from build123d import *

# Parameters (mm, degrees)
PAD_DEPTH       = 12
SKETCH004_R     = 8
SKETCH004_R_2   = 1.25
PAD001_DEPTH    = 5
SKETCH005_R     = 1.25
POCKET_DEPTH    = 8
PAD002_DEPTH    = 2
FILLET_R        = 2
CHAMFER_SIZE    = 0.6
CHAMFER001_SIZE = 0.5
FILLET001_R     = 2
FILLET002_R     = 2
CHAMFER002_SIZE = 0.6


with BuildPart() as part:
    # Sketch002 → Pad (new body)
    with BuildSketch(Plane.XY):
        with BuildLine():
            ThreePointArc((0, -7.5), (4.245918, -6.182409), (7, -2.692582))
            Line((7, 2.692582), (7, -2.692582))
            ThreePointArc((7, 2.692582), (4.245918, 6.182409), (0, 7.5))
            Line((-10.65, 5.289572), (0, 7.5))
            Line((-10.65, 5.289572), (-10.65, -5.289572))
            Line((-10.65, -5.289572), (0, -7.5))
        make_face()
        with BuildLine():
            ThreePointArc((-2.65, -1.702939), (3.15, 0), (-2.65, 1.702939))
            Line((-2.65, 1.702939), (-2.65, -1.702939))
        make_face(mode=Mode.SUBTRACT)
    extrude(amount=PAD_DEPTH)

    # Sketch004 → Pad001 (join)
    with BuildSketch(Plane.XY.offset(12)):
        with BuildLine():
            Line((-10.65, 8.5), (57.640793, 8.5))
            ThreePointArc((57.640793, -8.5), (85, 0), (57.640793, 8.5))
            Line((57.640793, -8.5), (-10.65, -8.5))
            Line((-10.65, -8.5), (-10.65, 8.5))
        make_face()
        with Locations((70, 0)):
            Circle(SKETCH004_R, mode=Mode.SUBTRACT)
        with Locations((64.25, 9.959292)):
            Circle(SKETCH004_R_2, mode=Mode.SUBTRACT)
        with Locations((81.5, 0)):
            Circle(SKETCH004_R_2, mode=Mode.SUBTRACT)
        with Locations((64.25, -9.959292)):
            Circle(SKETCH004_R_2, mode=Mode.SUBTRACT)
        with BuildLine():
            ThreePointArc((-2.65, -1.702939), (3.15, 0), (-2.65, 1.702939))
            Line((-2.65, 1.702939), (-2.65, -1.702939))
        make_face(mode=Mode.SUBTRACT)
    extrude(amount=PAD001_DEPTH)

    # Sketch005 (on Face1 of Pad001) → Pocket (cut)
    with BuildSketch(Plane(origin=(-10.65, 0, 0), x_dir=(0, -1, 0), z_dir=(-1, 0, 0))):
        with Locations((0, 14.5)):
            Circle(SKETCH005_R)
        with Locations((0, 8.5)):
            Circle(SKETCH005_R)
        with Locations((0, 2.5)):
            Circle(SKETCH005_R)
    extrude(amount=-POCKET_DEPTH, mode=Mode.SUBTRACT)

    # Sketch006 (on Face16 of Pocket) → Pad002 (join, symmetric)
    with BuildSketch(Plane(origin=(0, 0, 0), x_dir=(-1, 0, 0), z_dir=(0, 1, 0))):
        Polygon((-7, 0), (-55, 12), (-7, 12), align=None)
    extrude(amount=PAD002_DEPTH, both=True)

    # Fillet
    fillet_edges = [part.edges().sort_by_distance(p)[0] for p in [
        (-10.65, 8.5, 14.5),
        (-10.65, 5.289572, 6),
        (-10.65, -5.289572, 6),
        (-10.65, -8.5, 14.5),
    ]]
    fillet(fillet_edges, radius=FILLET_R)

    # Chamfer
    chamfer_edges = [part.edges().sort_by_distance(p)[0] for p in [
        (3.15, 0, 0),
        (-2.65, 0, 0),
    ]]
    chamfer(chamfer_edges, length=CHAMFER_SIZE)

    # Chamfer001
    chamfer001_edges = [part.edges().sort_by_distance(p)[0] for p in [
        (62, 0, 12),
    ]]
    chamfer(chamfer001_edges, length=CHAMFER001_SIZE)

    # Fillet001
    fillet001_edges = [part.edges().sort_by_distance(p)[0] for p in [
        (57.640793, 8.5, 14.5),
    ]]
    fillet(fillet001_edges, radius=FILLET001_R)

    # Fillet002
    fillet002_edges = [part.edges().sort_by_distance(p)[0] for p in [
        (57.640793, -8.5, 14.5),
    ]]
    fillet(fillet002_edges, radius=FILLET002_R)

    # Chamfer002
    chamfer002_edges = [part.edges().sort_by_distance(p)[0] for p in [
        (-10.65, 1.25, 2.5),
        (-10.65, 1.25, 8.5),
        (-10.65, 1.25, 14.5),
    ]]
    chamfer(chamfer002_edges, length=CHAMFER002_SIZE)


solid = part.part
Check sheet for the modelled part. Datum: model origin and axes. Units: mm. A direction names the side the tool comes from. Round coordinates to 2 decimals unless told otherwise and drop trailing zeros. Order: outer loops, then holes, each group sorted by start corner. A loop starts at its lowest first (then second) coordinate and runs counter-clockwise, first axis right, second up.
(1) Access from +Z, -Z, +X, -X, +Y, -Y to the whole of each face (thin tool, end or side, straight path). Record for faces 4 (the flat face through (24, 8.5, 14)), 5 (the flat face through (25, -2, 7)), 6 (the cylindrical face through (4.298, 6.146, 5.916)), 7 (the cylindrical face through (-10.213, 4.91, 6.084)).
(2) Cross-section at C-C, the plane x = 81.5. Enter the section's corners in (y, z), and give its area (3 significant figures).
(3) Cross-section at B-B, the plane z = 2.5. Enter the section's corners in (x, y).
(4) Draft check along X on faces 1 (the cylindrical face through (3.15, -0.11, 8.69)), 2 (the cylindrical face through (57.5, 8.7, 14.5)), 3 (the flat face through (24, -8.5, 14)). Enter one of: pulls with the +X half, pulls with the -X half, needs draft (parallel to the pull), parting line crosses it, or undercut.
(5) Scan lines: probe 1 along Z at (x, y) = (-6.25, 0); probe 2 along Y at (x, z) = (54, 13.5); probe 3 along Z at (x, y) = (34, -5). Record each from-to range of solid material in increasing order.
(6) Cross-section at D-D, the plane z = 14.5. Enter the section's corners in (x, y).
(7) Go/stop test with flat-tipped pins: P1, Ø10, axis at x = 20, y = 2, coming from the -Z side; P2, Ø10, axis at x = 0, z = 11.5, coming from the +Y side; P3, Ø5, axis at y = -10.5, z = 14.5, coming from the -X side. Record where each tip stops, or that it passes through.
(8) Cross-section at A-A, the plane x = 70. Enter the section's corners in (y, z).
Check sheet entries:
1. face 4: +Z, -Z, -X, +Y
1. face 5: -Z, +X, -Y
1. face 6: -Z, +X, +Y
1. face 7: -Z, -X, +Y
2. outline: (-9.63, 12) - (-1.25, 12) - (-1.25, 17) - (-9.63, 17) - close; (1.25, 12) - (9.63, 12) - (9.63, 17) - (1.25, 17) - close
2. area: 83.8 mm2
3. outline: (-10.65, -3.66) arc R2 ccw to (-9.06, -5.62) - (0, -7.5) arc R7.5 ccw to (7, -2.69) - (7, -2) - (17, -2) - (17, 2) - (7, 2) - (7, 2.69) arc R7.5 ccw to (0, 7.5) - (-9.06, 5.62) arc R2 ccw to (-10.65, 3.66) - (-10.65, 1.85) - (-10.05, 1.25) - (-2.65, 1.25) - (-2.65, 1.7) arc R3.15 cw (long way) to (-2.65, -1.7) - (-2.65, -1.25) - (-10.05, -1.25) - (-10.65, -1.85) - close
4. face 1: undercut
4. face 2: pulls with the -X half
4. face 3: needs draft
5. probe 1: z = 0 to 1.25, 3.75 to 7.25, 9.75 to 13.25, 15.75 to 17
5. probe 2: y = -8.5 to 8.5
5. probe 3: z = 12 to 17
6. outline: (-10.65, -6.5) arc R2 ccw to (-8.65, -8.5) - (56.63, -8.5) arc R2 cw to (58.2, -9.26) arc R15 ccw (long way) to (58.2, 9.26) arc R2 cw to (56.63, 8.5) - (-8.65, 8.5) arc R2 ccw to (-10.65, 6.5) - (-10.65, 1.85) - (-10.05, 1.25) - (-2.65, 1.25) - (-2.65, 1.7) arc R3.15 cw (long way) to (-2.65, -1.7) - (-2.65, -1.25) - (-10.05, -1.25) - (-10.65, -1.85) - close; hole circle Ø16 at (70, 0); hole circle Ø2.5 at (64.25, -9.96); hole circle Ø2.5 at (64.25, 9.96); hole circle Ø2.5 at (81.5, 0)
7. P1: stops at z = 2
7. P2: stops at y = 8.5
7. P3: stops at x = -9.97
8. outline: (-15, 12) - (-8.5, 12) - (-8, 12.5) - (-8, 17) - (-15, 17) - close; (8, 12.5) - (8.5, 12) - (15, 12) - (15, 17) - (8, 17) - close
